Source: CAD feature listing. Evaluate the final solid. Frame: model axes, mm. A direction names the side the tool comes from. Coordinates: 2 decimals unless noted, no trailing zeros. Order: outer loops, then holes, each group sorted by start corner. A loop starts at its lowest first (then second) coordinate and runs counter-clockwise, first axis right, second up. Notation, with made-up numbers: (-21, -26.5) -> (35, -26.5) arc R14 cw to (35, -13.5) -> close; hole circle Ø11 at (68, -38.75). An arc over 180 degrees is marked (long way). Write each question's results on one line, items separated by ' | '. Start each with the question number.
Autodesk Inventor part; units mm, degrees
ref_plane "РабПлоскость1" through (1.85, 0, 0) normal (1, 0, 0) x (0, 1, 0)
ref_plane "XZ Plane" through (0, 0, 0) normal (0, 1, 0) x (-1, 0, 0)
ref_plane "XY Plane" through (0, 0, 0) normal (0, 0, 1) x (1, 0, 0)
sketch "Эскиз1" plane through (0, 0, 0) normal (0, 1, 0) x (-1, 0, 0)
  circle A0 centre (0, 0) radius 3.75
  circle A1 centre (0, 0) radius 2.425
  circle A2 centre (0, 0) radius 1.5
  dimension "d0" = 4.85
  dimension "d1" = 7.5
  dimension "d2" = 3
extrude "Выдавливание1" add sketch "Эскиз1" along normal blind 12 contours A1
extrude "Выдавливание2" add sketch "Эскиз1" against normal blind 1.25 contours A0 | A1
ref_plane "РабПлоскость1" through (1.85, 0, 0) normal (1, 0, 0) x (0, 1, 0)
sketch "Эскиз2" plane through (1.85, 0, 0) normal (1, 0, 0) x (0, 1, 0)
  line L0 (12, -2.425) -> (12, 2.425)
  line L1 (0, -2.425) -> (0, 2.425)
  line L2 (12, -2.425) -> (12, 2.425)
  line L3 (0, -2.425) -> (0, 2.425)
  line L4 (12, 0) -> (9.575, 2.425)
  line L5 (0, 2.425) -> (12, 2.425)
  line L6 (12, 0) -> (15.4295, 0) construction
  line L7 (9.575, 2.425) -> (12, 2.425)
  point P0 (0, 0)
  dimension "d8" = 135
extrude "Выдавливание3" cut sketch "Эскиз2" along normal blind 10
properties part number "Штырь"
(1) Section D-D on y = 1.75. Return the cut outline in (x, z) (3 decimals).
(2) Section B-B on z = 1. Return the cut outline in (x, y), then the cut area to 3 significant figures.
(3) First-contact query: P1, Ø4, axis at y = 8.5, z = 2.5, coming from the -X side; P2, Ø4, axis at x = 1, z = -1, coming from the +Y side; P3, Ø0.5, axis at y = 11.5, z = 0.5, coming from the +X side. Flat tips, straight axial feed; report the tip coordinate or a pass-through.
(4) Reachability of faces 4 (the cylindrical face through (3.746, -0.616, 0.165)), 5 (the flat face through (2, 0, 2)), 6 (the flat face through (1.85, 11.6, 1.1)) from +Z, -Z, +X, -X, +Y, -Y: full face, straight path, thin tool, end or side. Return the list, or none.
(5) Draft query along X for faces 1 (the cylindrical face through (-2.313, 5.916, -0.728)), 2 (the cylindrical face through (1.5, 5.28, -0.07)), 3 (the flat face through (-2, 12, 0)). Return one class per face: released by +X, released by -X, zero draft, split by the parting line, or undercut.
(6) Section A-A on x = 0. Return the cut outline in (y, z) (3 decimals).
(7) Section C-C on x = -1. Return the cut outline in (y, z).
(8) Line query: L1, parallel to Z at x = 0, y = 1.5 (3 decimals); L2, parallel to Y at x = 0.25, z = -2.75; L3, parallel to Z at x = -0.5, y = 1. Output: solid intervals per line, ascending.
Results list:
1) outline: circle Ø4.85 at (0, 0); hole circle Ø3 at (0, 0)
2) outline: (-3.61, -1.25) -> (-1.12, -1.25) -> (-1.12, 12) -> (-2.21, 12) -> (-2.21, 0) -> (-3.61, 0) -> close; (1.12, -1.25) -> (3.61, -1.25) -> (3.61, 0) -> (2.21, 0) -> (2.21, 11) -> (1.85, 11) -> (1.85, 12) -> (1.12, 12) -> close | area: 32.1 mm²
3) P1: stops at x = -2.37 | P2: stops at y = 12 | P3: stops at x = 2.41
4) face 4: +Y, -Y | face 5: +Y | face 6: +Z, +X, +Y
5) face 1: split by the parting line | face 2: undercut | face 3: zero draft
6) outline: (-1.25, -3.75) -> (0, -3.75) -> (0, -2.425) -> (12, -2.425) -> (12, -1.5) -> (-1.25, -1.5) -> close; (-1.25, 1.5) -> (12, 1.5) -> (12, 2.425) -> (0, 2.425) -> (0, 3.75) -> (-1.25, 3.75) -> close
7) outline: (-1.25, -3.61) -> (0, -3.61) -> (0, -2.21) -> (12, -2.21) -> (12, -1.12) -> (-1.25, -1.12) -> close; (-1.25, 1.12) -> (12, 1.12) -> (12, 2.21) -> (0, 2.21) -> (0, 3.61) -> (-1.25, 3.61) -> close
8) L1: z = -2.425 to -1.5, 1.5 to 2.425 | L2: y = -1.25 to 0 | L3: z = -2.37 to -1.41, 1.41 to 2.37
